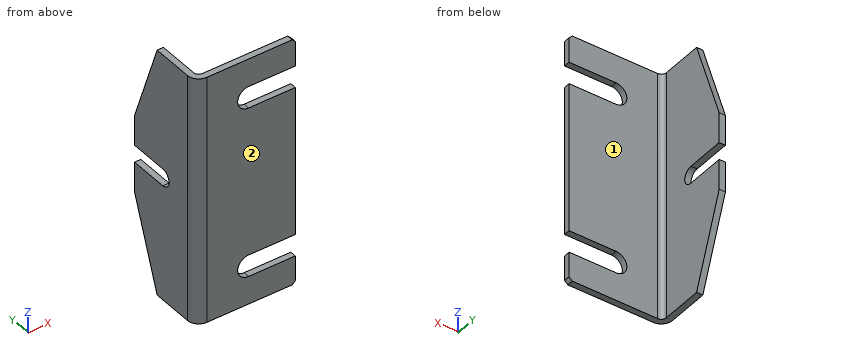
from build123d import *

# Parameters (mm, degrees)
BASE_FLANGE1_DEPTH = 80
CUT_EXTRUDE1_REACH = 113.803
CUT_EXTRUDE2_REACH = 113.803
CUT_EXTRUDE3_REACH = 113.803
CHAMFER1_SIZE      = 2


# Sheet-metal steps are written as plain solids
with BuildPart() as part:
    # Sketch1 → Base-Flange1 (new, symmetric)
    with BuildSketch(Plane.XY):
        with BuildLine():
            Line((60, 0), (3.175, 0))
            ThreePointArc((3.175, 0), (0.92993597, 0.92993597), (0, 3.175))
            Line((0, 3.175), (0, 50))
            Line((0, 50), (-4, 50))
            Line((-4, 50), (-4, 3.175))
            ThreePointArc((-4, 3.175), (-1.898491155, -1.898491155), (3.175, -4))
            Line((3.175, -4), (60, -4))
            Line((60, -4), (60, 0))
        make_face()
    extrude(amount=BASE_FLANGE1_DEPTH, both=True)

    # Sketch6 → Cut-Extrude1 (cut, up to next)
    with BuildSketch(Plane(origin=(0, 0, 0), x_dir=(0, 0, -1), z_dir=(1, 0, 0)), mode=Mode.PRIVATE) as cut_extrude1_sk1:
        with BuildLine():
            Line((5.5, 25), (5.5, 50))
            Line((5.5, 50), (-5.5, 50))
            Line((-5.5, 50), (-5.5, 25))
            ThreePointArc((-5.5, 25), (0, 19.5), (5.5, 25))
        make_face()
    cut_extrude1_tool1 = extrude(cut_extrude1_sk1.sketch, amount=-CUT_EXTRUDE1_REACH, mode=Mode.PRIVATE) & part.part
    add(cut_extrude1_tool1.solids().sort_by_distance((0, 35.314457, 0))[0], mode=Mode.SUBTRACT)

    # Sketch8 → Cut-Extrude2 (cut, up to next)
    with BuildSketch(Plane(origin=(0, 0, 0), x_dir=(0, 0, -1), z_dir=(1, 0, 0)), mode=Mode.PRIVATE) as cut_extrude2_sk1:
        Polygon((-80, 30), (-25, 50), (-80, 50), align=None)
    cut_extrude2_tool1 = extrude(cut_extrude2_sk1.sketch, amount=-CUT_EXTRUDE2_REACH, mode=Mode.PRIVATE) & part.part
    # Sketch8 → Cut-Extrude2 (cut, up to next)
    with BuildSketch(Plane(origin=(0, 0, 0), x_dir=(0, 0, -1), z_dir=(1, 0, 0)), mode=Mode.PRIVATE) as cut_extrude2_sk2:
        Polygon((25, 50), (80, 30), (80, 50), align=None)
    cut_extrude2_tool2 = extrude(cut_extrude2_sk2.sketch, amount=-CUT_EXTRUDE2_REACH, mode=Mode.PRIVATE) & part.part
    add(cut_extrude2_tool1.solids().sort_by_distance((0, 43.333333, 61.666667))[0], mode=Mode.SUBTRACT)
    add(cut_extrude2_tool2.solids().sort_by_distance((0, 43.333333, -61.666667))[0], mode=Mode.SUBTRACT)

    # Sketch9 → Cut-Extrude3 (cut, up to next)
    with BuildSketch(Plane(origin=(0, 0, 0), x_dir=(1, 0, 0), z_dir=(0, 1, 0)), mode=Mode.PRIVATE) as cut_extrude3_sk1:
        with BuildLine():
            Line((30, 62), (60, 62))
            Line((60, 62), (60, 48))
            Line((60, 48), (30, 48))
            ThreePointArc((30, 48), (23, 55), (30, 62))
        make_face()
    cut_extrude3_tool1 = extrude(cut_extrude3_sk1.sketch, amount=-CUT_EXTRUDE3_REACH, mode=Mode.PRIVATE) & part.part
    # Sketch9 → Cut-Extrude3 (cut, up to next)
    with BuildSketch(Plane(origin=(0, 0, 0), x_dir=(1, 0, 0), z_dir=(0, 1, 0)), mode=Mode.PRIVATE) as cut_extrude3_sk2:
        with BuildLine():
            Line((30, -48), (60, -48))
            Line((60, -48), (60, -62))
            Line((60, -62), (30, -62))
            ThreePointArc((30, -62), (23, -55), (30, -48))
        make_face()
    cut_extrude3_tool2 = extrude(cut_extrude3_sk2.sketch, amount=-CUT_EXTRUDE3_REACH, mode=Mode.PRIVATE) & part.part
    add(cut_extrude3_tool1.solids().sort_by_distance((42.216724, 0, -55))[0], mode=Mode.SUBTRACT)
    add(cut_extrude3_tool2.solids().sort_by_distance((42.216724, 0, 55))[0], mode=Mode.SUBTRACT)

    # Chamfer1
    chamfer1_edges = [part.edges().sort_by_distance(p)[0] for p in [
        (60, -2, 80),
        (60, -2, -80),
    ]]
    chamfer(chamfer1_edges, length=CHAMFER1_SIZE)


solid = part.part
Design review of the part built by this model. Coordinates are the model's own, in mm. Face numbers are marked on the shaded views. A direction names the side the tool comes from. Give positions to 0.01 mm unless a question says otherwise; leave off trailing zeros. Write each loop counter-clockwise with the first axis right and the second up, starting at its lowest first coordinate (ties: lowest second). Pieces come first, ordered by that corner, then holes. Notation, with made-up numbers: M 10.5,54.25 L 64.5,54.25 A9 cw 64.5,64.25 Z; hole C 85,22 d1. An arc over 180 degrees is marked long. Return JSON: item names as keys, results as strings. Group by question number.
Item 1: Take a section at A-A (x = 54.5). Give the boundary of the cut face in (y, z), plus the area to 3 significant figures.
Item 2: Clearance check with flat-ended pins moving along their axes: pin 1 Ø17 at (x, z) = (24.5, -27) entering from +Y; pin 2 Ø8 at (x, z) = (4.5, 46.5) entering from +Y; pin 3 Ø14 at (y, z) = (22, -25) entering from +X. State where each tip first meets the part, or that it passes through.
Item 3: Take a section at D-D (x = 17). Give the boundary of the cut face in (y, z).
Item 4: Take a section at B-B (z = 14.5). Give the boundary of the cut face in (x, y) (3 decimals).
Item 5: Tool access review of the marked faces 1 and 2: name each direction out of +Z, -Z, +X, -X, +Y, -Y from which nothing blocks a thin tool from reaching the whole face with its end or side.
Item 6: Take a section at C-C (y = 23). Give the boundary of the cut face in (x, z), plus the area to 3 significant figures.
Item 7: Wall thickness on line 1 along Y through (x, z) = (27.5, 73.5); line 2 along X through (y, z) = (1.5, 58): over which ranges is each line inside the solid? List them lowest first.
Return value:
{
 "1": {"outline": "M -4,-80 L 0,-80 L 0,-62 L -4,-62 Z; M -4,-48 L 0,-48 L 0,48 L -4,48 Z; M -4,62 L 0,62 L 0,80 L -4,80 Z", "area": "528 mm2"},
 "2": {"pin 1": "stops at y = 0", "pin 2": "stops at y = 1.46", "pin 3": "stops at x = 0"},
 "3": {"outline": "M -4,-80 L 0,-80 L 0,80 L -4,80 Z"},
 "4": {"outline": "M -4,3.175 A7.175 ccw 3.175,-4 L 60,-4 L 60,0 L 3.175,0 A3.175 cw 0,3.175 L 0,50 L -4,50 Z"},
 "5": {"face 1": "+Z, -Z, +X, +Y", "face 2": "+Z, -Z, +X, -X, -Y"},
 "6": {"outline": "M -4,-80 L 0,-80 L 0,-5.12 L -4,-5.12 Z; M -4,5.12 L 0,5.12 L 0,80 L -4,80 Z", "area": "599 mm2"},
 "7": {"line 1": "y = -4 to 0", "line 2": "x = -3.8 to 0.48"}
}
